Design review of the part built by this model. Coordinates are the model's own, in mm. A direction names the side the tool comes from. Give positions to 0.01 mm unless a question says otherwise; leave off trailing zeros. Order: outer loops, then holes, each group sorted by start corner. A loop starts at its lowest first (then second) coordinate and runs counter-clockwise, first axis right, second up. Notation, with made-up numbers: M 75,55.5 L 118,55.5 A17 cw 118,65.5 Z; hole C -27,52 d2. An arc over 180 degrees is marked long. Answer as a JSON object with one key per item and string values.
from build123d import *

# Parameters (mm, degrees)
EXTRUDE_583_DEPTH              = 5
SKETCH_2_W                     = 10
SKETCH_2_H                     = 30
EXTRUDE_642_DEPTH              = 5
CHAMFER_690_SIZE               = 1.5
CHAMFER_690_OF_MIRROR_757_SIZE = 1.5


with BuildPart() as part:
    # ｽｹｯﾁ1 → Extrude 583 (new, symmetric)
    with BuildSketch(Plane(origin=(0, 0, 0), x_dir=(0, 0, -1), z_dir=(1, 0, 0))):
        with BuildLine():
            Line((75.5, 0), (105, 0))
            Line((105, 0), (105, 94))
            Line((105, 94), (-105, 94))
            Line((-105, 94), (-105, 0))
            Line((-105, 0), (-75.5, 0))
            ThreePointArc((-75.5, 0), (0, 75.5), (75.5, 0))
        make_face()
    extrude(amount=EXTRUDE_583_DEPTH, both=True)

    # ｽｹｯﾁ2 → Extrude 642 (add, symmetric)
    with BuildSketch(Plane(origin=(0, 0, 0), x_dir=(0, 0, -1), z_dir=(1, 0, 0))):
        with Locations((-110, 45)):
            Rectangle(SKETCH_2_W, SKETCH_2_H)
    extrude_642 = extrude(amount=EXTRUDE_642_DEPTH, both=True)

    # Chamfer 690
    chamfer_690_edges = [part.edges().sort_by_distance(p)[0] for p in [
        (0, 60, 115),
        (0, 30, 115),
    ]]
    chamfer(chamfer_690_edges, length=CHAMFER_690_SIZE)

    # Mirror 757: Extrude 642 across plane
    add(extrude_642.mirror(Plane.XY))

    # Chamfer 690 of Mirror 757
    chamfer_690_of_mirror_757_edges = [part.edges().sort_by_distance(p)[0] for p in [
        (0, 60, -115),
        (0, 30, -115),
    ]]
    chamfer(chamfer_690_of_mirror_757_edges, length=CHAMFER_690_OF_MIRROR_757_SIZE)


solid = part.part
(1) To check wall thickness, follow L1, parallel to Y at x = 4.75, z = 1.5; L2, parallel to Z at x = -4, y = 86; L3, parallel to Z at x = 1, y = 34. State the ranges of each line that lie inside material, in increasing order. Write a range as from..to.
Checked values:
{"L1": "y = 75.49..94", "L2": "z = -105..105", "L3": "z = -115..-67.41, 67.41..115"}
(2) We need section A-A (y = 50). Write out the cut boundary in (x, z), plus the area to 3 significant figures.
Checked values:
{"outline": "M -5,-115 L 5,-115 L 5,-56.57 L -5,-56.57 Z; M -5,56.57 L 5,56.57 L 5,115 L -5,115 Z", "area": "1,170 mm^2"}
(3) We need section D-D (y = 23). Write out the cut boundary in (x, z), plus the area to 3 significant figures.
Checked values:
{"outline": "M -5,-105 L 5,-105 L 5,-71.91 L -5,-71.91 Z; M -5,71.91 L 5,71.91 L 5,105 L -5,105 Z", "area": "662 mm^2"}
(4) Tool access review of faces 4 (the flat face through (0, 77, -105)), 5 (the flat face through (0, 77, 105)), 6 (the flat face through (0, 15, 105)): name each direction out of +Z, -Z, +X, -X, +Y, -Y from which nothing blocks a thin tool from reaching the whole face with its end or side.
Checked values:
{"face 4": "-Z, +X, -X, +Y", "face 5": "+Z, +X, -X, +Y", "face 6": "+Z, +X, -X, -Y"}
(5) We need section C-C (z = 0). Write out the cut boundary in (x, y).
Checked values:
{"outline": "M -5,75.5 L 5,75.5 L 5,94 L -5,94 Z"}
(6) Draft analysis for pull direction Z (two halves, no side actions). For faces 1 (the cylindrical face through (0.07, 75.48, 1.66)), 2 (the flat face through (0, 30, -109)), 3 (the flat face through (0, 15, -105)), state which applies: +Z half, -Z half, draft (parallel to the pull), parting line (faces both ways), or undercut.
Checked values:
{"face 1": "undercut", "face 2": "draft", "face 3": "-Z half"}
(7) Insertion check: pin 1 (2.5 mm diameter, centred on x = -2, z = 107.5, fed in from +Y); pin 2 (6 mm diameter, centred on x = -4, z = 21, fed in from -Y); pin 3 (2.5 mm diameter, centred on x = -1.5, z = -110.5, fed in from -Y). Each pin has a flat end and moves straight along its axis. Give the tip position at first contact, or say it passes through.
Checked values:
{"pin 1": "stops at y = 60", "pin 2": "stops at y = 71.58", "pin 3": "stops at y = 30"}
(8) We need section B-B (x = -0.75). Write out the cut boundary in (y, z).
Checked values:
{"outline": "M 0,-105 L 30,-105 L 30,-113.5 L 31.5,-115 L 58.5,-115 L 60,-113.5 L 60,-105 L 94,-105 L 94,105 L 60,105 L 60,113.5 L 58.5,115 L 31.5,115 L 30,113.5 L 30,105 L 0,105 L 0,75.5 A75.5 cw 0,-75.5 Z"}
